Verification items for the finished model (mm, model axes). A direction names the side the tool comes from. Give positions to 0.01 mm unless a question says otherwise; leave off trailing zeros. Write each loop counter-clockwise with the first axis right and the second up, starting at its lowest first coordinate (ties: lowest second). Pieces come first, ordered by that corner, then holes. Notation, with made-up numbers: M 29.25,20 L 66.25,20 A15 cw 66.25,27 Z; hole C 59.25,57 d6. An arc over 180 degrees is marked long. Write item = value, one per line.
Solid Edge part; units mm, degrees
sketch "Sketch1" plane through (0, 0, 0) normal (0, -1, 0) x (1, 0, 0)
  arc A0 (0, 10) -> (3, 7.58) centre (0, 6.9305) cw
  line L0 (3, 7.58) -> (3, 7.5)
  line L1 (3, 7.5) -> (2.9202, 7.5058)
  line L2 (2.9202, 7.5058) -> (2.5, 5)
  line L3 (1.5, 5) -> (2.5, 5)
  line L4 (1.5, 0) -> (1.5, 5)
  line L5 (0, 0) -> (1.5, 0)
  line L6 (0, 0) -> (0, 10)
revolve "RevolvedProtrusion1" add sketch "Sketch1" angle 360 about axis through (0, 0, 0) along (0, 0, 1)
properties material "Tantalum"
1) Cross-section at C-C on z = 1.25. Record the boundary of the cut face in (x, y).
From the geometry:
outline = C 0,0 d3
2) Material ranges on probe 1 along X at (y, z) = (-0.2, 2); probe 2 along X at (y, z) = (-1.1, 3.5); probe 3 along Z at (x, y) = (0.55, -1.7), recorded low to high. Write a range as from..to.
From the geometry:
probe_1 = -1.49..1.49
probe_2 = -1.02..1.02
probe_3 = 5..9.43
3) Cross-section at D-D on z = 9. Record the boundary of the cut face in (x, y), plus the area to 3 significant figures.
From the geometry:
outline = C 0,0 d4.53
area = 16.1 mm^2
4) Depth check by flat-ended pin: P1, Ø1.5, axis at x = -1, z = 7, coming from the -Y side; P2, Ø3, axis at y = 2.5, z = 1.5, coming from the +X side. Enter the tip coordinate at first touch or a pass-through.
From the geometry:
P1 = -2.97
P2 = 1.12
5) Cross-section at A-A on x = 0. Record the boundary of the cut face in (y, z), plus the area to 3 significant figures.
From the geometry:
outline = M -3,7.5 L -2.92,7.51 L -2.5,5 L -1.5,5 L -1.5,0 L 1.5,0 L 1.5,5 L 2.5,5 L 2.92,7.51 L 3,7.5 L 3,7.58 A3.07 ccw -3,7.58 Z
area = 39.9 mm^2
6) Tool access check on faces 1 (the cylindrical face through (-1.5, 0.07, 2.54)), 2 (the flat face through (0, 0, 0)). Record the directions out of +Z, -Z, +X, -X, +Y, -Y that give a thin tool (end or side, any length) a straight path to the whole face; none if there is none.
From the geometry:
face_1 = -Z
face_2 = -Z, +X, -X, +Y, -Y
